Check sheet for the modelled part. Datum: model origin and axes. Units: mm. A direction names the side the tool comes from. Round coordinates to 2 decimals unless told otherwise and drop trailing zeros. Loops run counter-clockwise (first coordinate to the right, second up) from the corner with the lowest first, then second, coordinate; pieces in that order, holes last. Notation, with made-up numbers: (-31.5, -38) - (19.5, -38) arc R21 ccw to (19.5, -32) - close; hole circle Ø7 at (39, -8.5). An arc over 180 degrees is marked (long way). Return JSON: item names as keys, results as strings.
from build123d import *

# Parameters (mm, degrees)
SKETCH_1_W          = 209.185842875
SKETCH_1_H          = 10
SKETCH_1_R          = 1.6
EXTRUDE_1_DEPTH     = 10
SKETCH_2_W          = 8
SKETCH_2_H          = 8
CUT_EXTRUDE_1_DEPTH = 327.126841673


with BuildPart() as part:
    # ｽｹｯﾁ1 → ﾎﾞｽ - 押し出し1 (new body)
    with BuildSketch(Plane.XY):
        with Locations((-467.701812763, 245)):
            Rectangle(SKETCH_1_W, SKETCH_1_H)
        with Locations((-368.108891325, 245)):
            Circle(SKETCH_1_R, mode=Mode.SUBTRACT)
        with Locations((-567.2947342, 244.999999998)):
            Circle(SKETCH_1_R, mode=Mode.SUBTRACT)
    extrude(amount=EXTRUDE_1_DEPTH)

    # ｽｹｯﾁ2 → ｶｯﾄ - 押し出し1 (cut, through all)
    with BuildSketch(Plane.ZY.offset(572.2947342)):
        with Locations((5, 245)):
            Rectangle(SKETCH_2_W, SKETCH_2_H)
    extrude(amount=-CUT_EXTRUDE_1_DEPTH, mode=Mode.SUBTRACT)


solid = part.part
Q1. Sectioned sample at A-A (z = 2.5). Enter the section's corners in (x, y), plus the area to 3 significant figures.
Answer key:
{"outline": "(-572.29, 240) - (-363.11, 240) - (-363.11, 241) - (-572.29, 241) - close; (-572.29, 249) - (-363.11, 249) - (-363.11, 250) - (-572.29, 250) - close", "area": "418 mm²"}
Q2. Scan lines: probe 1 along X at (y, z) = (245, 9.65); probe 2 along Z at (x, y) = (-515, 246.75); probe 3 along Y at (x, z) = (-438.5, 6.75). Record each from-to range of solid material in increasing order. Write a range as [from, to].
Answer key:
{"probe 1": "x = [-572.29, -568.89], [-565.69, -369.71], [-366.51, -363.11]", "probe 2": "z = [0, 1], [9, 10]", "probe 3": "y = [240, 241], [249, 250]"}
Q3. Tool access check on faces 5 (the face through (-469, 241, 5)), 6 (the face through (-469, 245, 0)). Record the directions out of +Z, -Z, +X, -X, +Y, -Y that give a thin tool (end or side, any length) a straight path to the whole face; none if there is none.
Answer key:
{"face 5": "+X, -X", "face 6": "-Z, +X, -X, +Y, -Y"}
Q4. Draft check along Y on faces 1 (the face through (-469, 240, 5)), 2 (the face through (-572.295, 249.4, 4.9)), 3 (the face through (-568.893, 245.07, 0.493)), 4 (the face through (-469, 250, 5)). Enter one of: released by +Y, released by -Y, zero draft, split by the parting line, or undercut.
Answer key:
{"face 1": "released by -Y", "face 2": "zero draft", "face 3": "undercut", "face 4": "released by +Y"}
Q5. Sectioned sample at C-C (x = -401). Enter the section's corners in (y, z).
Answer key:
{"outline": "(240, 0) - (250, 0) - (250, 10) - (240, 10) - close; hole (241, 1) - (249, 1) - (249, 9) - (241, 9) - close"}
Q6. Sectioned sample at B-B (y = 245). Enter the section's corners in (x, z), plus the area to 3 significant figures.
Answer key:
{"outline": "(-572.29, 0) - (-568.89, 0) - (-568.89, 1) - (-572.29, 1) - close; (-572.29, 9) - (-568.89, 9) - (-568.89, 10) - (-572.29, 10) - close; (-565.69, 0) - (-369.71, 0) - (-369.71, 1) - (-565.69, 1) - close; (-565.69, 9) - (-369.71, 9) - (-369.71, 10) - (-565.69, 10) - close; (-366.51, 0) - (-363.11, 0) - (-363.11, 1) - (-366.51, 1) - close; (-366.51, 9) - (-363.11, 9) - (-363.11, 10) - (-366.51, 10) - close", "area": "406 mm²"}
Q7. Depth check by flat-ended pin: P1, Ø2.5, axis at x = -451.5, y = 246, coming from the -Z side. Enter the tip coordinate at first touch or a pass-through.
Answer key:
{"P1": "stops at z = 0"}
